from build123d import *

# Parameters (mm, degrees)
SKETCH1_R           = 4
BOSS_EXTRUDE1_DEPTH = 1
CHAMFER1_SIZE       = 0.5
CHAMFER1_SIZE2      = 1
CUT_EXTRUDE1_DEPTH  = 0.9
SKETCH3_R           = 1.5
BOSS_EXTRUDE2_DEPTH = 6


with BuildPart() as part:
    # Sketch1 → Boss-Extrude1 (new body)
    with BuildSketch(Plane(origin=(0, 0, 0), x_dir=(1, 0, 0), z_dir=(0, 1, 0))):
        with Locations(Location((0, 0, 0), (0, 0, 270))):
            Circle(SKETCH1_R)
    extrude(amount=BOSS_EXTRUDE1_DEPTH)

    # Chamfer1
    chamfer1_edges = [part.edges().sort_by_distance(p)[0] for p in [
        (0, 1, -4),
    ]]
    chamfer1_side = [part.faces().sort_by_distance(p)[0] for p in [
        (0, 0.5, -4),
    ]]
    chamfer(chamfer1_edges, length=CHAMFER1_SIZE, length2=CHAMFER1_SIZE2, reference=chamfer1_side[0])

    # Sketch2 → Cut-Extrude1 (cut)
    with BuildSketch(Plane(origin=(0, 1, 0), x_dir=(1, 0, 0), z_dir=(0, 1, 0))):
        Polygon((0.88903539, 0.736851009), (-0.193613998, 1.138352737), (-1.082649387, 0.401501728), (-0.88903539, -0.736851009), (0.193613998, -1.138352737), (1.082649387, -0.401501728), align=None)
    extrude(amount=-CUT_EXTRUDE1_DEPTH, mode=Mode.SUBTRACT)

    # Sketch3 → Boss-Extrude2 (add)
    with BuildSketch(Plane.XZ):
        with Locations(Location((0, 0, 0), (0, 0, 90))):
            Circle(SKETCH3_R)
    extrude(amount=BOSS_EXTRUDE2_DEPTH)


solid = part.part
Design review of the part built by this model. Coordinates are the model's own, in mm. A direction names the side the tool comes from. Give positions to 0.01 mm unless a question says otherwise; leave off trailing zeros. Write each loop counter-clockwise with the first axis right and the second up, starting at its lowest first coordinate (ties: lowest second). Pieces come first, ordered by that corner, then holes. Notation, with made-up numbers: M 62,41 L 78,41 A17 cw 78,58 Z; hole C -9.75,-28.75 d1. An arc over 180 degrees is marked long. Answer as a JSON object with one key per item and string values. Group by question number.
1) Tool access review of faces 4 (the face through (0, -6, 0)), 5 (the face through (0, 0.1, 0)): name each direction out of +Z, -Z, +X, -X, +Y, -Y from which nothing blocks a thin tool from reaching the whole face with its end or side.
2) We need section B-B (x = 0). Give the boundary of the cut face in (y, z).
3) We need section C-C (y = -2.25). Give the boundary of the cut face in (x, z), and give its area (3 significant figures).
4) Clearance check with a flat-ended pin moving along its axis: pin 1 Ø1 at (y, z) = (-4, 0) entering from +X. State where the tip first meets the part, or that it passes through.
5) For line 1 along Y through (x, z) = (2, -0.75); line 2 along X through (y, z) = (-2, 0); line 3 along Z through (x, y) = (-0.5, -4), list the stretches that pass through material, from the lowest coordinate up.
6) We need section A-A (z = 0). Give the boundary of the cut face in (x, y), and give its area (3 significant figures).
7) Mouldability with a two-part tool opening along X and no side actions: class faces 1 (the face through (-0.355, 0.556, 0.935)), 2 (the face through (0, 0, 2)), 3 (the face through (-0.45, -2.96, 1.43)) as released by +X, released by -X, zero draft, split by the parting line, or undercut.
Answer key:
{
 "1": {"face 4": "+Z, -Z, +X, -X, -Y", "face 5": "+Y"},
 "2": {"outline": "M -6,-1.5 L 0,-1.5 L 0,-4 L 0.5,-4 L 1,-3 L 1,-1.07 L 0.1,-1.07 L 0.1,1.07 L 1,1.07 L 1,3 L 0.5,4 L 0,4 L 0,1.5 L -6,1.5 Z"},
 "3": {"outline": "C 0,0 d3", "area": "7.07 mm²"},
 "4": {"pin 1": "stops at x = 1.5"},
 "5": {"line 1": "y = 0 to 1", "line 2": "x = -1.5 to 1.5", "line 3": "z = -1.41 to 1.41"},
 "6": {"outline": "M -4,0 L -1.5,0 L -1.5,-6 L 1.5,-6 L 1.5,0 L 4,0 L 4,0.5 L 3,1 L 1.01,1 L 1.01,0.1 L -1.01,0.1 L -1.01,1 L -3,1 L -4,0.5 Z", "area": "23.7 mm²"},
 "7": {"face 1": "undercut", "face 2": "zero draft", "face 3": "split by the parting line"}
}
